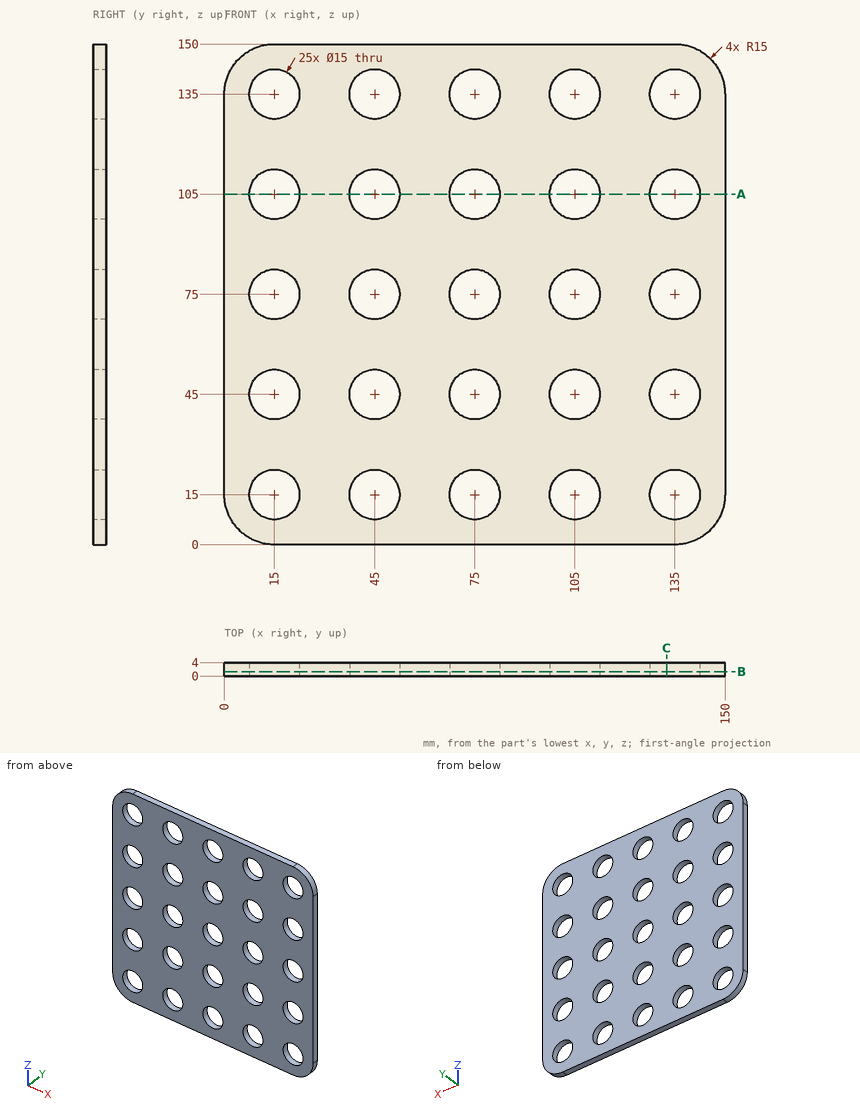
Print and shaded views of the part. All mm, measured from the part's lowest x, y and z. Coordinates: 2 decimals unless noted, no trailing zeros. Order: outer loops, then holes, each group sorted by start corner. A loop starts at its lowest first (then second) coordinate and runs counter-clockwise, first axis right, second up. Notation, with made-up numbers: (30.5, 60.25) -> (83.5, 60.25) arc R32 ccw to (83.5, 98.25) -> close; hole circle Ø9 at (44.25, 49.25). An arc over 180 degrees is marked (long way). Use one line per item in the form item = value. Start each with the question number.
1) Drop a flat-ended pin along its axis: pin 1 (9 mm diameter, centred on x = 75, z = 15, fed in from +Y). Give the stop position or say it passes through.
2) Drill centre lines: L1, parallel to X at y = 1.05, z = 75; L2, parallel to X at y = 1.8, z = 16.5. Where is each one in solid material? Low to high. Write a range as [from, to].
3) Band-saw the part on B-B on y = 1.3. State how many separate pieces and enclosed holes the cut face has, then the cut area to 3 significant figures.
4) Band-saw the part on A-A on z = 105. Give the cut face in (x, y).
5) Band-saw the part on C-C on x = 132.5. Give the cut face in (y, z), then the cut area to 3 significant figures.
Entries:
q1.pin_1 = through
q2.L1 = [0, 7.5], [22.5, 37.5], [52.5, 67.5], [82.5, 97.5], [112.5, 127.5], [142.5, 150]
q2.L2 = [0, 7.65], [22.35, 37.65], [52.35, 67.65], [82.35, 97.65], [112.35, 127.65], [142.35, 150]
q3.separate_pieces = 1
q3.enclosed_holes = 25
q3.area = 17,900 mm2
q4.outline = (0, 0) -> (7.5, 0) -> (7.5, 4) -> (0, 4) -> close; (22.5, 0) -> (37.5, 0) -> (37.5, 4) -> (22.5, 4) -> close; (52.5, 0) -> (67.5, 0) -> (67.5, 4) -> (52.5, 4) -> close; (82.5, 0) -> (97.5, 0) -> (97.5, 4) -> (82.5, 4) -> close; (112.5, 0) -> (127.5, 0) -> (127.5, 4) -> (112.5, 4) -> close; (142.5, 0) -> (150, 0) -> (150, 4) -> (142.5, 4) -> close
q5.outline = (0, 0) -> (4, 0) -> (4, 7.93) -> (0, 7.93) -> close; (0, 22.07) -> (4, 22.07) -> (4, 37.93) -> (0, 37.93) -> close; (0, 52.07) -> (4, 52.07) -> (4, 67.93) -> (0, 67.93) -> close; (0, 82.07) -> (4, 82.07) -> (4, 97.93) -> (0, 97.93) -> close; (0, 112.07) -> (4, 112.07) -> (4, 127.93) -> (0, 127.93) -> close; (0, 142.07) -> (4, 142.07) -> (4, 150) -> (0, 150) -> close
q5.area = 317 mm2
